Can you work these out from the model? Positions are in its coordinate system, mm. Face numbers are marked on the shaded views. A direction names the side the tool comes from. Give positions to 0.01 mm unless a question says otherwise; leave off trailing zeros. Loops run counter-clockwise (first coordinate to the right, second up) from the corner with the lowest first, then second, coordinate; pieces in that order, holes last. Notation, with made-up numbers: (86.5, -30) - (99.5, -30) arc R29 ccw to (99.5, 3) - close; hole circle Ø5 at (-25, -28.5). An arc over 180 degrees is marked (long way). Answer as a JSON object with one key per item and string values.
```python
from build123d import *

# Parameters (mm, degrees)
SKETCH1_W               = 70
SKETCH1_H               = 15
BASE_FLANGE1_DEPTH      = 2
EDGE_FLANGE1_DEPTH      = 20
EDGE_FLANGE1_START      = 2
EDGE_FLANGE1_PROFILE_R  = 2.25
EDGE_FLANGE1_FLAT_DEPTH = 2
SKETCH18_R              = 2.1
CUT_EXTRUDE1_DEPTH      = 10


# Sheet-metal steps are written as plain solids
with BuildPart() as part:
    # Sketch1 → Base-Flange1 (new body)
    with BuildSketch(Plane(origin=(0, 0, 0), x_dir=(1, 0, 0), z_dir=(0, 1, 0))):
        Rectangle(SKETCH1_W, SKETCH1_H)
    extrude(amount=-BASE_FLANGE1_DEPTH)

    # Edge-Flange1 bend section (across the edge) → Edge-Flange1 (add)
    with BuildSketch(Plane(origin=(10, 0, -8.2366), x_dir=(0, 0, 1), z_dir=(-1, 0, 0))):
        with BuildLine():
            Line((-2, 0.7366), (0, 0.7366))
            ThreePointArc((0, 0.7366), (0.215745145, 0.215745145), (0.7366, 0))
            Line((0.7366, 0), (0.7366, -2))
            ThreePointArc((0.7366, -2), (-1.198468417, -1.198468417), (-2, 0.7366))
        make_face()
    extrude(amount=EDGE_FLANGE1_DEPTH)

    # Edge-Flange1 profile (on flange) → Edge-Flange1 flat (add)
    with BuildSketch(Plane(origin=(0, 0, -8.2366), x_dir=(-1, 0, 0), z_dir=(0, 0, -1)).offset(EDGE_FLANGE1_START)):
        Polygon((-10, 0.7366), (10, 0.7366), (10, 54.366187709), (35, 54.366187709), (35, 116.622772523), (-35, 116.622772523), (-35, 54.366187709), (-10, 54.366187709), align=None)
        with Locations((25, 60.5)):
            Circle(EDGE_FLANGE1_PROFILE_R, mode=Mode.SUBTRACT)
        with BuildLine():
            Line((29.55, 98.490926284), (29.55, 72.509073716))
            ThreePointArc((29.55, 72.509073716), (22.825059318, 62.674940682), (12.990926284, 55.95))
            Line((12.990926284, 55.95), (0.75, 55.95))
            Line((0.75, 55.95), (0.75, 73.527045436))
            ThreePointArc((0.75, 73.527045436), (10.389206213, 79.501788996), (10.74388281, 90.836958229))
            Line((10.74388281, 90.836958229), (28.322327677, 100.985878105))
            ThreePointArc((28.322327677, 100.985878105), (28.963041516, 99.751627692), (29.55, 98.490926284))
        make_face(mode=Mode.SUBTRACT)
        with Locations((-25, 60.5)):
            Circle(EDGE_FLANGE1_PROFILE_R, mode=Mode.SUBTRACT)
        with BuildLine():
            Line((-0.75, 55.95), (-12.990926284, 55.95))
            ThreePointArc((-12.990926284, 55.95), (-22.825059318, 62.674940682), (-29.55, 72.509073716))
            Line((-29.55, 72.509073716), (-29.55, 98.490926284))
            ThreePointArc((-29.55, 98.490926284), (-28.963041516, 99.751627692), (-28.322327677, 100.985878105))
            Line((-28.322327677, 100.985878105), (-10.74388281, 90.836958229))
            ThreePointArc((-10.74388281, 90.836958229), (-10.389206213, 79.501788996), (-0.75, 73.527045436))
            Line((-0.75, 73.527045436), (-0.75, 55.95))
        make_face(mode=Mode.SUBTRACT)
        with Locations((25, 110.5)):
            Circle(EDGE_FLANGE1_PROFILE_R, mode=Mode.SUBTRACT)
        with BuildLine():
            Line((-10.156894371, 91.883700942), (-27.727157775, 102.027897248))
            ThreePointArc((-27.727157775, 102.027897248), (-21.374853973, 109.688474184), (-12.990926284, 115.05))
            Line((-12.990926284, 115.05), (12.990926284, 115.05))
            ThreePointArc((12.990926284, 115.05), (21.262202003, 109.787557137), (27.572327677, 102.28491621))
            Line((27.572327677, 102.28491621), (9.99388281, 92.135996335))
            ThreePointArc((9.99388281, 92.135996335), (-0.150187994, 97.495481839), (-10.156894371, 91.883700942))
        make_face(mode=Mode.SUBTRACT)
        with Locations((-25, 110.5)):
            Circle(EDGE_FLANGE1_PROFILE_R, mode=Mode.SUBTRACT)
    extrude(amount=-EDGE_FLANGE1_FLAT_DEPTH)

    # Sketch18 → Cut-Extrude1 (cut)
    with BuildSketch(Plane(origin=(0, 0, 0), x_dir=(1, 0, 0), z_dir=(0, 1, 0))):
        with Locations(Location((-25, 0, 0), (0, 0, 270))):
            Circle(SKETCH18_R)
        with Locations(Location((25, 0, 0), (0, 0, 270))):
            Circle(SKETCH18_R)
    extrude(amount=-CUT_EXTRUDE1_DEPTH, mode=Mode.SUBTRACT)


solid = part.part
```
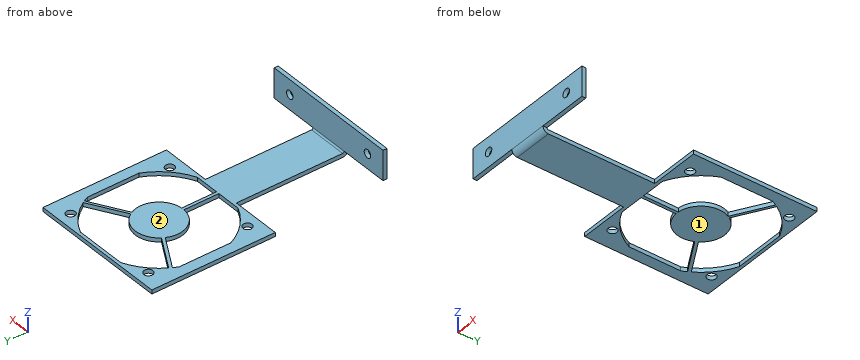
1) I need wall thicknesses on L1, parallel to X at y = -1, z = 0; L2, parallel to Y at x = -25, z = -9.4; L3, parallel to Y at x = -29.5, z = -6. Which ranges of each line are inside material? Lowest first, please.
Check sheet entries:
{"L1": "-35 to -27.1, -22.9 to 22.9, 27.1 to 35", "L2": "54.37 to 58.25, 62.75 to 65.08, 99.07 to 100.8, 105.92 to 108.25, 112.75 to 116.62", "L3": "-2 to 0"}
2) Imagine slicing it at A-A on z = 0. Write out the boundary of the cut face in (x, y), and give its area (3 significant figures).
Check sheet entries:
{"outline": "(-35, -2) - (-27.1, -2) - (-27.1, 0) - (-35, 0) - close; (-22.9, -2) - (22.9, -2) - (22.9, 0) - (-22.9, 0) - close; (27.1, -2) - (35, -2) - (35, 0) - (27.1, 0) - close", "area": "123 mm2"}
3) Imagine slicing it at D-D on y = 110.5. Write out the boundary of the cut face in (x, z).
Check sheet entries:
{"outline": "(-35, -10.24) - (-27.25, -10.24) - (-27.25, -8.24) - (-35, -8.24) - close; (-22.75, -10.24) - (-20.42, -10.24) - (-20.42, -8.24) - (-22.75, -8.24) - close; (20.42, -10.24) - (22.75, -10.24) - (22.75, -8.24) - (20.42, -8.24) - close; (27.25, -10.24) - (35, -10.24) - (35, -8.24) - (27.25, -8.24) - close"}
4) Which directions (+Z, -Z, +X, -X, +Y, -Y) give clear straight access to the entire face, cutting with the end or side of a thin tool? Please do the marked faces 1 and 2.
Check sheet entries:
{"face 1": "-Z, +X, -X, +Y, -Y", "face 2": "+Z, +X, -X, +Y"}
5) Imagine slicing it at B-B on y = 60.5. Write out the boundary of the cut face in (x, z), and give its area (3 significant figures).
Check sheet entries:
{"outline": "(-35, -10.24) - (-27.25, -10.24) - (-27.25, -8.24) - (-35, -8.24) - close; (-22.75, -10.24) - (-20.42, -10.24) - (-20.42, -8.24) - (-22.75, -8.24) - close; (-0.75, -10.24) - (0.75, -10.24) - (0.75, -8.24) - (-0.75, -8.24) - close; (20.42, -10.24) - (22.75, -10.24) - (22.75, -8.24) - (20.42, -8.24) - close; (27.25, -10.24) - (35, -10.24) - (35, -8.24) - (27.25, -8.24) - close", "area": "43.3 mm2"}
6) Imagine slicing it at C-C on x = 8.5. Write out the boundary of the cut face in (y, z).
Check sheet entries:
{"outline": "(-2, -7.5) arc R2.74 ccw to (0.74, -10.24) - (55.95, -10.24) - (55.95, -8.24) - (0.74, -8.24) arc R0.74 cw to (0, -7.5) - (0, 7.5) - (-2, 7.5) - close; (77.03, -10.24) - (93.97, -10.24) - (93.97, -8.24) - (77.03, -8.24) - close; (115.05, -10.24) - (116.62, -10.24) - (116.62, -8.24) - (115.05, -8.24) - close"}
7) I'm going to push flat-ended pins straight in: P1, Ø5, axis at x = -2, y = 60.5, coming from the -Z side; P2, Ø21, axis at x = 1.5, y = 33, coming from the +Z side; P3, Ø1, axis at x = -23.5, z = -9, coming from the -Y side; P4, Ø3.5, axis at x = -25, z = 0, coming from the -Y side. Where does each tip first touch, or does it pass through?
Check sheet entries:
{"P1": "z = -10.24", "P2": "z = -8.24", "P3": "y = 54.37", "P4": "through"}
